from build123d import *

# Parameters (mm, degrees)
SKETCH1_W                                       = 324
SKETCH1_H                                       = 40
BOSS_EXTRUDE1_DEPTH                             = 10
G1_4_TAPPED_HOLE1_D                             = 6
CSK_FOR_M3_COUNTERSUNK_FLAT_HEAD1_D             = 3.4
CSK_FOR_M3_COUNTERSUNK_FLAT_HEAD1_CSINK_D       = 6.3
CSK_FOR_M3_COUNTERSUNK_FLAT_HEAD1_CSINK_ANGLE   = 90
SKETCH9_W                                       = 10
SKETCH9_H                                       = 324
BOSS_EXTRUDE2_DEPTH                             = 80
CSK_FOR_M3_COUNTERSUNK_FLAT_HEAD2_D             = 3.4
CSK_FOR_M3_COUNTERSUNK_FLAT_HEAD2_DEPTH         = 11.5
CSK_FOR_M3_COUNTERSUNK_FLAT_HEAD2_CSINK_D       = 6.3
CSK_FOR_M3_COUNTERSUNK_FLAT_HEAD2_CSINK_ANGLE   = 90
CSK_FOR_M3_COUNTERSUNK_FLAT_HEAD2_TIP           = 1.021463052
M3X0_5_TAPPED_HOLE1_AT_2_COUNT                  = 2
M3X0_5_TAPPED_HOLE1_AT_2_PITCH                  = 30
M3X0_5_TAPPED_HOLE1_AT_3_COUNT                  = 2
M3X0_5_TAPPED_HOLE1_AT_3_PITCH                  = 60
M3X0_5_TAPPED_HOLE1_AT_4_COUNT                  = 2
M3X0_5_TAPPED_HOLE1_AT_4_PITCH                  = 90
SKETCH14_W                                      = 8
SKETCH14_H                                      = 324
CUT_EXTRUDE1_DEPTH                              = 1
CSK_FOR_M3_FLAT_HEAD_MACHINE_SCREW1_D           = 3.4
CSK_FOR_M3_FLAT_HEAD_MACHINE_SCREW1_CSINK_D     = 6.3
CSK_FOR_M3_FLAT_HEAD_MACHINE_SCREW1_CSINK_ANGLE = 90
LPATTERN1_COUNT                                 = 7
LPATTERN1_PITCH                                 = 42
SKETCH18_R                                      = 12.5
SKETCH18_R_2                                    = 2.5
MOD_CUT_DEPTH                                   = 191.641023917


with BuildPart() as part:
    # Sketch1 → Boss-Extrude1 (new body)
    with BuildSketch(Plane(origin=(0, 0, 0), x_dir=(0, 0, -1), z_dir=(1, 0, 0))):
        Rectangle(SKETCH1_W, SKETCH1_H)
    extrude(amount=BOSS_EXTRUDE1_DEPTH)

    # G1/4 Tapped Hole1 (through all)
    with Locations(Plane(origin=(0, -10, 0), x_dir=(0, 0, -1), z_dir=(-1, 0, 0))):
        with Locations((0, 0), (154, -7)):
            Hole(G1_4_TAPPED_HOLE1_D / 2)

    # CSK for M3 Countersunk Flat Head1 (through all)
    with Locations(Plane(origin=(0, -10, -10), x_dir=(0, 0, -1), z_dir=(-1, 0, 0))):
        with Locations((0, 0)):
            csk_for_m3_countersunk_flat_head1 = CounterSinkHole(CSK_FOR_M3_COUNTERSUNK_FLAT_HEAD1_D / 2, CSK_FOR_M3_COUNTERSUNK_FLAT_HEAD1_CSINK_D / 2, counter_sink_angle=CSK_FOR_M3_COUNTERSUNK_FLAT_HEAD1_CSINK_ANGLE)

    # Mirror1: CSK for M3 Countersunk Flat Head1 across plane
    add(csk_for_m3_countersunk_flat_head1.mirror(Plane.XY), mode=Mode.SUBTRACT)

    # Sketch9 → Boss-Extrude2 (add)
    with BuildSketch(Plane.XZ.offset(20)):
        with Locations((5, 0)):
            Rectangle(SKETCH9_W, SKETCH9_H)
    extrude(amount=BOSS_EXTRUDE2_DEPTH)

    # CSK for M3 Countersunk Flat Head2
    with Locations(Plane(origin=(10, -96, 125), x_dir=(0, 0, 1), z_dir=(1, 0, 0))):
        with Locations((0, 0), (-50, 0), (-100, 0), (-150, 0), (-200, 0), (-250, 0)):
            CounterSinkHole(CSK_FOR_M3_COUNTERSUNK_FLAT_HEAD2_D / 2, CSK_FOR_M3_COUNTERSUNK_FLAT_HEAD2_CSINK_D / 2, depth=CSK_FOR_M3_COUNTERSUNK_FLAT_HEAD2_DEPTH, counter_sink_angle=CSK_FOR_M3_COUNTERSUNK_FLAT_HEAD2_CSINK_ANGLE)
            with Locations((0, 0, -(CSK_FOR_M3_COUNTERSUNK_FLAT_HEAD2_DEPTH + CSK_FOR_M3_COUNTERSUNK_FLAT_HEAD2_TIP / 2))):  # 118° drill point
                Cone(0, CSK_FOR_M3_COUNTERSUNK_FLAT_HEAD2_D / 2, CSK_FOR_M3_COUNTERSUNK_FLAT_HEAD2_TIP, mode=Mode.SUBTRACT)

    # Sketch13 → M3x0.5 Tapped Hole1 (revolve, cut)
    with BuildSketch(Plane(origin=(5, 5, 162), x_dir=(0, -1, 0), z_dir=(1, 0, 0))):
        Polygon((0, 0), (0, 12.251075774), (1.25, 11.5), (1.25, 0), align=None)
    m3x0_5_tapped_hole1 = revolve(axis=Axis((5, 5, 168.35), (0, 0, -1)), mode=Mode.SUBTRACT)

    # M3x0.5 Tapped Hole1 at 2: M3x0.5 Tapped Hole1 ×2
    with Locations(*[(0, -i * M3X0_5_TAPPED_HOLE1_AT_2_PITCH, 0) for i in range(1, M3X0_5_TAPPED_HOLE1_AT_2_COUNT)]):
        add(m3x0_5_tapped_hole1, mode=Mode.SUBTRACT)

    # M3x0.5 Tapped Hole1 at 3: M3x0.5 Tapped Hole1 ×2
    with Locations(*[(0, -i * M3X0_5_TAPPED_HOLE1_AT_3_PITCH, 0) for i in range(1, M3X0_5_TAPPED_HOLE1_AT_3_COUNT)]):
        add(m3x0_5_tapped_hole1, mode=Mode.SUBTRACT)

    # M3x0.5 Tapped Hole1 at 4: M3x0.5 Tapped Hole1 ×2
    with Locations(*[(0, -i * M3X0_5_TAPPED_HOLE1_AT_4_PITCH, 0) for i in range(1, M3X0_5_TAPPED_HOLE1_AT_4_COUNT)]):
        add(m3x0_5_tapped_hole1, mode=Mode.SUBTRACT)

    # Mirror2: M3x0.5 Tapped Hole1 across plane
    add(m3x0_5_tapped_hole1.mirror(Plane.XY), mode=Mode.SUBTRACT)

    # Mirror2 copy 1 sketch → Mirror2 copy 1 (revolve, cut)
    with BuildSketch(Plane(origin=(5, -25, -162), x_dir=(0, -1, 0), z_dir=(1, 0, 0))):
        Polygon((0, 0), (0, -12.251075774), (1.25, -11.5), (1.25, 0), align=None)
    revolve(axis=Axis((5, -25, -168.35), (0, 0, -1)), mode=Mode.SUBTRACT)

    # Mirror2 copy 2 sketch → Mirror2 copy 2 (revolve, cut)
    with BuildSketch(Plane(origin=(5, -55, -162), x_dir=(0, -1, 0), z_dir=(1, 0, 0))):
        Polygon((0, 0), (0, -12.251075774), (1.25, -11.5), (1.25, 0), align=None)
    revolve(axis=Axis((5, -55, -168.35), (0, 0, -1)), mode=Mode.SUBTRACT)

    # Mirror2 copy 3 sketch → Mirror2 copy 3 (revolve, cut)
    with BuildSketch(Plane(origin=(5, -85, -162), x_dir=(0, -1, 0), z_dir=(1, 0, 0))):
        Polygon((0, 0), (0, -12.251075774), (1.25, -11.5), (1.25, 0), align=None)
    revolve(axis=Axis((5, -85, -168.35), (0, 0, -1)), mode=Mode.SUBTRACT)

    # Sketch14 → Cut-Extrude1 (cut)
    with BuildSketch(Plane(origin=(0, 20, 0), x_dir=(1, 0, 0), z_dir=(0, 1, 0))):
        with Locations((6, 0)):
            Rectangle(SKETCH14_W, SKETCH14_H)
    extrude(amount=-CUT_EXTRUDE1_DEPTH, mode=Mode.SUBTRACT)

    # CSK for M3 Flat Head Machine Screw1 (through all)
    with Locations(Plane(origin=(0, -25, -126), x_dir=(0, 0, -1), z_dir=(-1, 0, 0))):
        with Locations((0, 0)):
            csk_for_m3_flat_head_machine_screw1 = CounterSinkHole(CSK_FOR_M3_FLAT_HEAD_MACHINE_SCREW1_D / 2, CSK_FOR_M3_FLAT_HEAD_MACHINE_SCREW1_CSINK_D / 2, counter_sink_angle=CSK_FOR_M3_FLAT_HEAD_MACHINE_SCREW1_CSINK_ANGLE)

    # LPattern1: CSK for M3 Flat Head Machine Screw1 ×7
    with Locations(*[(0, 0, i * LPATTERN1_PITCH) for i in range(1, LPATTERN1_COUNT)]):
        add(csk_for_m3_flat_head_machine_screw1, mode=Mode.SUBTRACT)

    # Sketch18 → mod_cut (cut, through all)
    with BuildSketch(Plane.ZY):
        with Locations((-137, -65)):
            Circle(SKETCH18_R)
        with Locations((-105, -65)):
            Circle(SKETCH18_R_2)
        with Locations((-35, -65)):
            Circle(SKETCH18_R_2)
        with Locations((35, -65)):
            Circle(SKETCH18_R_2)
        with Locations((105, -65)):
            Circle(SKETCH18_R_2)
    extrude(amount=-MOD_CUT_DEPTH, mode=Mode.SUBTRACT)


solid = part.part
Read the model definition and answer for the solid it produces. Units are mm, in the model's axes. A direction names the side the tool comes from. Coordinates: 2 decimals unless noted, no trailing zeros. Return JSON: item names as keys, results as strings.
(1) Which of the six approach directions +Z, -Z, +X, -X, +Y, -Y give full straight-line access (tool end or side, diameter ignored) to faces 1 (the flat face through (6, 19, -2)), 2 (the cylindrical face through (4.93, -61.245, -125.077))?
Answers below:
{"face 1": "+Z, -Z, +X, +Y", "face 2": "+X, -X"}
(2) Each of these flat-tipped pins is pushed along its axis until it touches: P1, Ø2, axis at y = -25, z = -84, coming from the -X side; P2, Ø4.5, axis at y = -25, z = -126, coming from the -X side; P3, Ø1.5, axis at x = 5, y = -85, coming from the +Z side; P4, Ø4, axis at y = -96, z = 25, coming from the +X side. Where does it stop, or does it pass through?
Answers below:
{"P1": "through", "P2": "x = 0.9", "P3": "z = 150.2", "P4": "x = 8.85"}
(3) Consider line 1 along Y through (x, z) = (5, -158.25); line 2 along Y through (x, z) = (4.5, 126); line 3 along Z through (x, y) = (3.25, -64). Determine where each line is inside the solid, lowest interval first. Write a range as from..to.
Answers below:
{"line 1": "-100..-86.25, -83.75..-56.25, -53.75..-26.25, -23.75..3.75, 6.25..19", "line 2": "-100..-97.37, -94.63..-26.7, -23.3..19", "line 3": "-162..-149.46, -124.54..-107.29, -102.71..-37.29, -32.71..32.71, 37.29..102.71, 107.29..162"}
(4) For a pull along Z with two mould halves and no side action, classify faces 3 (the flat face through (5, -100, 2)), 4 (the flat face through (5, -39, 162)), 5 (the cylindrical face through (5.07, -3.9, -151.14)), 6 (the flat face through (5, -39, -162)) as pulls with the +Z half, pulls with the -Z half, needs draft (parallel to the pull), parting line crosses it, or undercut.
Answers below:
{"face 3": "needs draft", "face 4": "pulls with the +Z half", "face 5": "undercut", "face 6": "pulls with the -Z half"}
